from build123d import *

# Parameters (mm, degrees)
BOX001_W     = 114.5
BOX001_H     = 112.5
BOX001_DEPTH = 32
BOX_W        = 122.5
BOX_H        = 120.5
BOX_DEPTH    = 25
FILLET_R     = 31
FILLET001_R  = 31
FILLET002_R  = 31
FILLET003_R  = 31
FILLET004_R  = 34
FILLET005_R  = 34
FILLET006_R  = 34


with BuildPart() as cubo001:
    # Box001 → Box001 (new body)
    with BuildSketch(Plane(origin=(4, 4, 0), x_dir=(1, 0, 0), z_dir=(0, 0, 1))):
        with Locations((57.25, 56.25)):
            Rectangle(BOX001_W, BOX001_H)
    extrude(amount=BOX001_DEPTH)


with BuildPart() as fillet006:
    # Box → Box (new body)
    with BuildSketch(Plane.XY):
        with Locations((61.25, 60.25)):
            Rectangle(BOX_W, BOX_H)
    extrude(amount=BOX_DEPTH)

    # Cut: cut Cubo001
    add(cubo001.part, mode=Mode.SUBTRACT)

    # Fillet
    fillet_edges = [fillet006.edges().sort_by_distance(p)[0] for p in [
        (4, 116.5, 12.5),
    ]]
    fillet(fillet_edges, radius=FILLET_R)

    # Fillet001
    fillet001_edges = [fillet006.edges().sort_by_distance(p)[0] for p in [
        (118.5, 116.5, 12.5),
    ]]
    fillet(fillet001_edges, radius=FILLET001_R)

    # Fillet002
    fillet002_edges = [fillet006.edges().sort_by_distance(p)[0] for p in [
        (4, 4, 12.5),
    ]]
    fillet(fillet002_edges, radius=FILLET002_R)

    # Fillet003
    fillet003_edges = [fillet006.edges().sort_by_distance(p)[0] for p in [
        (118.5, 4, 12.5),
    ]]
    fillet(fillet003_edges, radius=FILLET003_R)

    # Fillet004
    fillet004_edges = [fillet006.edges().sort_by_distance(p)[0] for p in [
        (0, 120.5, 12.5),
    ]]
    fillet(fillet004_edges, radius=FILLET004_R)

    # Fillet005
    fillet005_edges = [fillet006.edges().sort_by_distance(p)[0] for p in [
        (122.5, 120.5, 12.5),
    ]]
    fillet(fillet005_edges, radius=FILLET005_R)

    # Fillet006
    fillet006_edges = [fillet006.edges().sort_by_distance(p)[0] for p in [
        (122.5, 0, 12.5),
    ]]
    fillet(fillet006_edges, radius=FILLET006_R)


solid = fillet006.part
Geometry check sheet. Reference: the model listing, model coordinates, mm. A direction names the side the tool comes from. Give positions to 0.01 mm unless a question says otherwise; leave off trailing zeros. Loops run counter-clockwise (first coordinate to the right, second up) from the corner with the lowest first, then second, coordinate; pieces in that order, holes last.
(1) Thickness scan on L1, parallel to Y at x = 53, z = 23.5; L2, parallel to X at y = 49.5, z = 1.5; L3, parallel to Y at x = 10.5, z = 21.5. Record the ranges inside material, lowest first.
From the geometry:
L1: y = 0 to 4, 116.5 to 120.5
L2: x = 0 to 4, 118.5 to 122.5
L3: y = 0 to 16.01, 104.49 to 111.07
(2) Section check C-C on x = 104. Record the cut outline in (y, z).
From the geometry:
outline: (3.74, 0) - (8.76, 0) - (8.76, 25) - (3.74, 25) - close; (111.74, 0) - (116.76, 0) - (116.76, 25) - (111.74, 25) - close
(3) Depth check by flat-ended pin: pin 1 Ø8 at (y, z) = (108.5, 3.5) entering from -X; pin 2 Ø4 at (x, z) = (101.5, 3.5) entering from -Y. Enter the tip coordinate at first touch or a pass-through.
From the geometry:
pin 1: stops at x = 5.16
pin 2: stops at y = 1.83
(4) Set-up check for faces 1 (the flat face through (2, 56, 25)), 2 (the flat face through (4, 60, 12)): record each of +Z, -Z, +X, -X, +Y, -Y from which the full face is reachable in a straight line by a thin tool's end or side.
From the geometry:
face 1: +Z, +X, -X, +Y, -Y
face 2: +Z, -Z
(5) Release check for a two-part mould opening along Y. For faces 3 (the flat face through (0, 43, 12)), 4 (the flat face through (61, 4, 12)), 5 (the cylindrical face through (112.28, 110.8, 12.68)) record: released by +Y, released by -Y, zero draft, split by the parting line, or undercut.
From the geometry:
face 3: zero draft
face 4: undercut
face 5: released by +Y
(6) Section check A-A on y = 71.5. Record the cut outline in (x, z).
From the geometry:
outline: (0, 0) - (4, 0) - (4, 25) - (0, 25) - close; (118.5, 0) - (122.5, 0) - (122.5, 25) - (118.5, 25) - close
(7) Section check B-B on z = 13.25. Record the cut outline in (x, y).
From the geometry:
outline: (0, 0) - (88.5, 0) arc R34 ccw to (122.5, 34) - (122.5, 86.5) arc R34 ccw to (88.5, 120.5) - (34, 120.5) arc R34 ccw to (0, 86.5) - close; hole (4, 35) arc R31 ccw to (35, 4) - (87.5, 4) arc R31 ccw to (118.5, 35) - (118.5, 85.5) arc R31 ccw to (87.5, 116.5) - (35, 116.5) arc R31 ccw to (4, 85.5) - close
